Input: dimensioned drawing with shaded views. Units: mm. Origin: part minimum x, y, z. A direction names the side the tool comes from. Give positions to 0.01 mm unless a question says otherwise; leave off trailing zeros. Loops run counter-clockwise (first coordinate to the right, second up) from the corner with the lowest first, then second, coordinate; pieces in that order, holes last. Notation, with made-up numbers: (-33.75, 39.5) -> (-21.75, 39.5) arc R27 cw to (-21.75, 75.5) -> close; hole circle Ø6 at (-32.75, 52.25). An arc over 180 degrees is marked (long way). Answer as a JSON object with one key per item and string values.
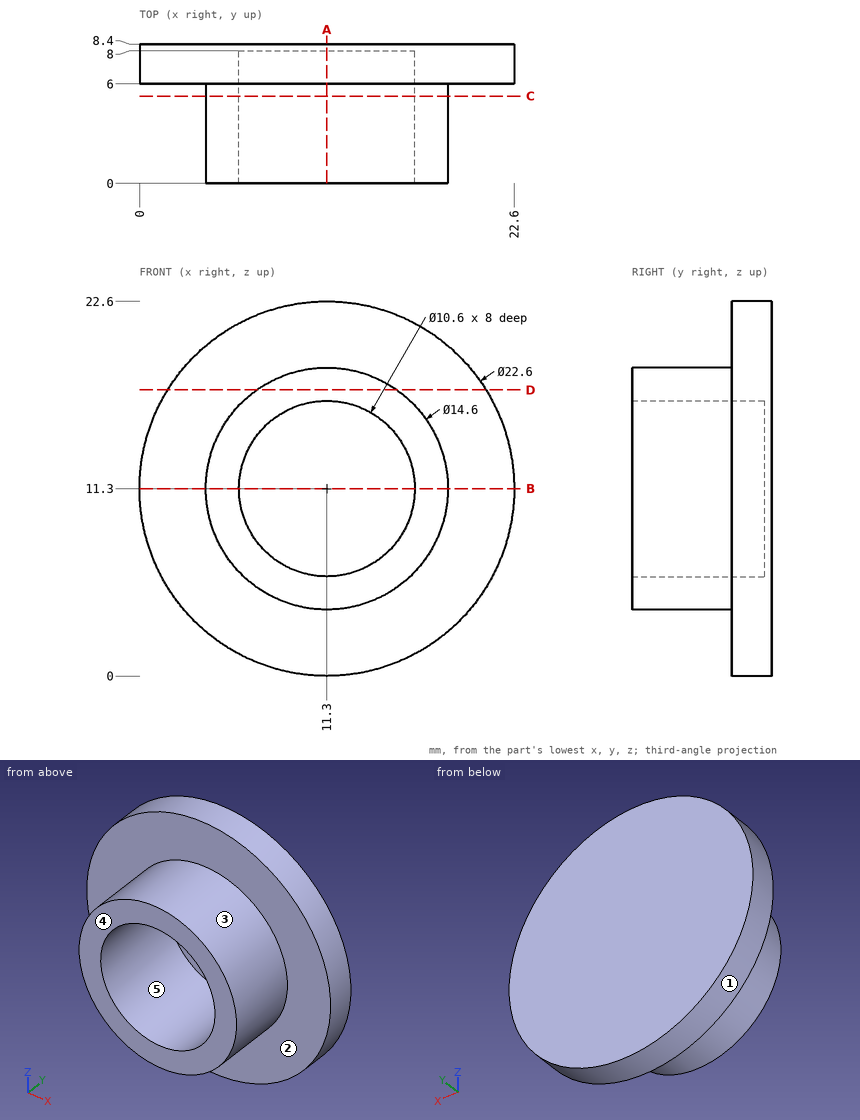
Q1. Section A-A, the plane x = 11.3. Return the cut outline in (y, z), then the cut area to 3 significant figures.
Evaluation:
{"outline": "(0, 4) -> (6, 4) -> (6, 0) -> (8.4, 0) -> (8.4, 22.6) -> (6, 22.6) -> (6, 18.6) -> (0, 18.6) -> (0, 16.6) -> (8, 16.6) -> (8, 6) -> (0, 6) -> close", "area": "57.0 mm2"}
Q2. Access query for the marked faces 1 and 2. Directions: +Z, -Z, +X, -X, +Y, -Y. A direction counts if a zero-diameter tool reaches every point of the face in a straight line with its end or side. Return the directions, or none.
Evaluation:
{"face 1": "+Y, -Y", "face 2": "-Y"}
Q3. Section D-D, the plane z = 17.25. Return the cut outline in (x, y).
Evaluation:
{"outline": "(1.69, 6) -> (7.07, 6) -> (7.07, 0) -> (15.53, 0) -> (15.53, 6) -> (20.91, 6) -> (20.91, 8.4) -> (1.69, 8.4) -> close"}
Q4. Draft query along Z for the marked faces 3, 4 and 5. Return one class per face: +Z half, -Z half, draft (parallel to the pull), parting line (faces both ways), or undercut.
Evaluation:
{"face 3": "parting line", "face 4": "draft", "face 5": "undercut"}
Q5. Pin query (flat end, axial travel): pin 1 (5 mm diameter, centred on y = 3, z = 3, fed in from -X); pin 2 (1.5 mm diameter, centred on x = 5.5, z = 19, fed in from -Y); pin 3 (1.5 mm diameter, centred on x = 9.5, y = 3.5, fed in from -Z). Return the tip coordinate at first contact, or that it passes through.
Evaluation:
{"pin 1": "stops at x = 6.87", "pin 2": "stops at y = 6", "pin 3": "stops at z = 4.08"}
Q6. Ray query, line 1 along Z through (x, y) = (11.3, 4.25); line 2 along X through (y, z) = (6.25, 11.3). Return the intervals inside material, ascending.
Evaluation:
{"line 1": "z = 4 to 6, 16.6 to 18.6", "line 2": "x = 0 to 6, 16.6 to 22.6"}
Q7. Section B-B, the plane z = 11.3. Return the cut outline in (x, y), then the cut area to 3 significant figures.
Evaluation:
{"outline": "(0, 6) -> (4, 6) -> (4, 0) -> (6, 0) -> (6, 8) -> (16.6, 8) -> (16.6, 0) -> (18.6, 0) -> (18.6, 6) -> (22.6, 6) -> (22.6, 8.4) -> (0, 8.4) -> close", "area": "57.0 mm2"}
Q8. Section C-C, the plane y = 5.25. Return the cut outline in (x, z), then the cut area to 3 significant figures.
Evaluation:
{"outline": "circle Ø14.6 at (11.3, 11.3); hole circle Ø10.6 at (11.3, 11.3)", "area": "79.2 mm2"}
